Study the drawing (mm; zero at the part's minimum x, y, z) and answer. A direction names the side the tool comes from. Round coordinates to 2 decimals unless told otherwise and drop trailing zeros. Loops run counter-clockwise (first coordinate to the right, second up) from the corner with the lowest first, then second, coordinate; pieces in that order, holes last. Notation, with made-up numbers: M 14,36 L 45,36 A8 cw 45,41 Z; hole C 65,40 d4. An arc over 180 degrees is marked long. Put each result on its own line as item: value. Start each with the question number.
(1) Determine the mould class of the marked faces 1, 2 and 3 for opening direction X: released by +X, released by -X, zero draft, split by the parting line, or undercut.
(2) Straight lines are drawn through the part: line 1 (Z direction, x = 25.5, y = 58.5) (1 decimal); line 2 (Z direction, x = 14.5, y = 58.5) (1 decimal); line 3 (Y direction, x = 21.5, z = 34). For each, find the intervals that lie inside material, in ascending order.
(3) Section A-A, the plane x = 5 is taken. Determine the outline of the cut face in (y, z).
(4) Flat-ended cylindrical pins translate along their axes: P1, Ø0.7, axis at x = 23.5, y = 58.5, coming from the -Z side (1 decimal); P2, Ø1, axis at y = 19, z = 49, coming from the -X side (3 decimals); P3, Ø2, axis at x = 20.5, y = 58, coming from the +Z side (1 decimal); P4, Ø11.5, axis at y = 47.752, z = 47.752, coming from the +X side. Find the tip coordinate at first contact, or state that the pin passes through.
(5) Which of the six approach directions +Z, -Z, +X, -X, +Y, -Y give full straight-line access (tool end or side, diameter ignored) to the marked faces 4 and 5?
(6) Section B-B, the plane x = 16.5 is taken. Determine the outline of the cut face in (y, z).
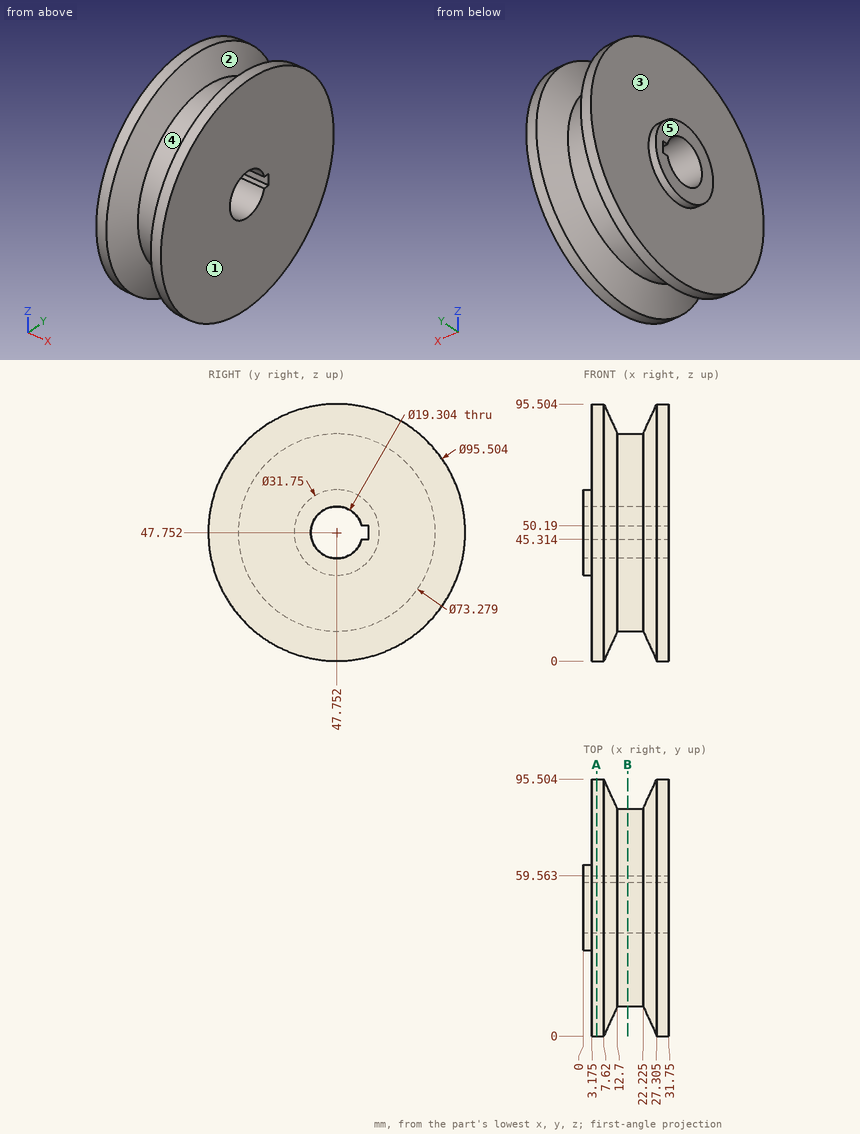
Recorded:
1. face 1: released by +X
1. face 2: undercut
1. face 3: released by -X
2. line 1: z = 5.3 to 45.3, 50.2 to 90.2
2. line 2: z = 12.7 to 45.3, 50.2 to 82.8
2. line 3: y = 13.79 to 81.71
3. outline: C 47.75,47.75 d95.5; hole M 57.09,45.31 L 59.56,45.31 L 59.56,50.19 L 57.09,50.19 A9.65 ccw long Z
4. P1: stops at z = 9
4. P2: stops at x = 3.175
4. P3: stops at z = 83.2
4. P4: passes through
5. face 4: none
5. face 5: +Z, -Z, -X, +Y, -Y
6. outline: C 47.75,47.75 d73.28; hole M 57.09,45.31 L 59.56,45.31 L 59.56,50.19 L 57.09,50.19 A9.65 ccw long Z
